Read the model definition and answer for the solid it produces. Units are mm, in the model's axes. A direction names the side the tool comes from. Give positions to 0.01 mm unless a question says otherwise; leave off trailing zeros. Loops run counter-clockwise (first coordinate to the right, second up) from the corner with the lowest first, then second, coordinate; pieces in that order, holes last.
(1) Straight lines are drawn through the part: probe 1 along Y at (x, z) = (33, 6.25); probe 2 along X at (y, z) = (75, 4.5); probe 3 along Y at (x, z) = (47.5, 7.25). For each, find the intervals that lie inside material, in ascending order.
(2) Find section A-A, the plane x = -33. Write down the section's boundary in (y, z), then the cut area to 3 significant figures.
(3) Determine the mould class of faces 4 (the face through (124.74, 4.88, 3.94)), 5 (the face through (100.9, 80.03, 3.94)), 6 (the face through (81, 61, 8)), 7 (the face through (-76.754, 45, 4)) for opening direction X: pulls with the +X half, pulls with the -X half, needs draft (parallel to the pull), parting line crosses it, or undercut.
(4) Which of the six approach directions +Z, -Z, +X, -X, +Y, -Y give full straight-line access (tool end or side, diameter ignored) to faces 1 (the face through (206.47, 43.18, 3.94)), 2 (the face through (-16, 49.585, 4)), 3 (the face through (-98.699, 11, 4))?
(5) Find section B-B, the plane y = -12.5. Write down the section's boundary in (x, z), then the cut area to 3 significant figures.
(6) Find section C-C, the plane z = 3.5. State how many separate pieces and enclosed holes the cut face has, then the cut area to 3 significant figures.
(7) Each of these flat-tipped pins is pushed along its axis until it touches: P1, Ø4, axis at y = 23.5, z = 4.5, coming from the +X side; P2, Ø3, axis at y = 74, z = 3, coming from the -X side; P3, Ø2.5, axis at x = -95, z = 4.5, coming from the +Y side. Where does it stop, or does it pass through?
```python
from build123d import *

# Parameters (mm, degrees)
ESQUISSE1_R        = 1.5
BOSS_EXTRU_1_DEPTH = 8


with BuildPart() as part:
    # Esquisse1 → Boss.-Extru.1 (new body)
    with BuildSketch(Plane.XY):
        Polygon((43.238760989, 49.585106383), (-75.988646329, 49.585106383), (-76.753762562, 49.585106383), (-76.753762562, 40.085106383), (2.011353671, 40.085106383), (50.71612997, 40.085106383), (151.689760112, 98.382258927), (214.4831558, 115.207698591), (229.494660416, 59.184000666), (174.076924484, 44.334863077), (66.257183131, -17.914893617), (-98.698564415, -17.914893617), (-98.698564415, 40.655573641), (-94.860830925, 40.655573641), (-92.861789188, 40.655573641), (-92.861789188, 49.585106383), (-94.860830925, 49.585106383), (-95.960869343, 49.585106383), (-101.253762562, 44.292213164), (-101.253762562, 35.79522772), (-101.253762562, -22.122000398), (-95.960869343, -27.414893617), (63.734552111, -27.414893617), (73.191845678, -24.880819443), (177.743787613, 35.482272378), (236.017194438, 51.096584676), (239.759835125, 57.579028501), (228.577013006, 99.31388882), (223.918643626, 116.699160027), (222.600104344, 121.736116557), (216.144691957, 125.488029577), (211.058449045, 124.125174896), (148.022896982, 107.234849626), (52.44172146, 52.051032209), align=None)
        with Locations((-95.753762562, -21.914893617)):
            Circle(ESQUISSE1_R, mode=Mode.SUBTRACT)
        with Locations((67.039694146, -20.835264486)):
            Circle(ESQUISSE1_R, mode=Mode.SUBTRACT)
        with Locations((-95.753762562, 44.085106383)):
            Circle(ESQUISSE1_R, mode=Mode.SUBTRACT)
        with Locations((-66.988646329, 44.085106383)):
            Circle(ESQUISSE1_R, mode=Mode.SUBTRACT)
        with Locations((49.263745973, 45.505477252)):
            Circle(ESQUISSE1_R, mode=Mode.SUBTRACT)
        with Locations((175.637377655, 40.567595866)):
            Circle(ESQUISSE1_R, mode=Mode.SUBTRACT)
        with Locations((234.393639901, 56.355573542)):
            Circle(ESQUISSE1_R, mode=Mode.SUBTRACT)
        with Locations((150.12930694, 102.149526137)):
            Circle(ESQUISSE1_R, mode=Mode.SUBTRACT)
        with Locations((217.363403759, 120.120565138)):
            Circle(ESQUISSE1_R, mode=Mode.SUBTRACT)
    extrude(amount=BOSS_EXTRU_1_DEPTH)


solid = part.part
```
Entries:
1. probe 1: y = -27.41 to -17.91, 40.09 to 49.59
1. probe 2: x = 92.19 to 111.19, 225.26 to 235.09
1. probe 3: y = -27.41 to -17.91, 40.09 to 50.73
2. outline: (-27.41, 0) - (-17.91, 0) - (-17.91, 8) - (-27.41, 8) - close; (40.09, 0) - (49.59, 0) - (49.59, 8) - (40.09, 8) - close
2. area: 152 mm2
3. face 4: pulls with the +X half
3. face 5: pulls with the -X half
3. face 6: needs draft
3. face 7: undercut
4. face 1: +Z, -Z, +X, -Y
4. face 2: +Z, -Z, -X, +Y
4. face 3: +Z, -Z
5. outline: (-101.25, 0) - (-98.7, 0) - (-98.7, 8) - (-101.25, 8) - close; (75.64, 0) - (94.64, 0) - (94.64, 8) - (75.64, 8) - close
5. area: 172 mm2
6. separate pieces: 1
6. enclosed holes: 9
6. area: 7,090 mm2
7. P1: stops at x = 160.45
7. P2: stops at x = 87.86
7. P3: stops at y = 49.59
